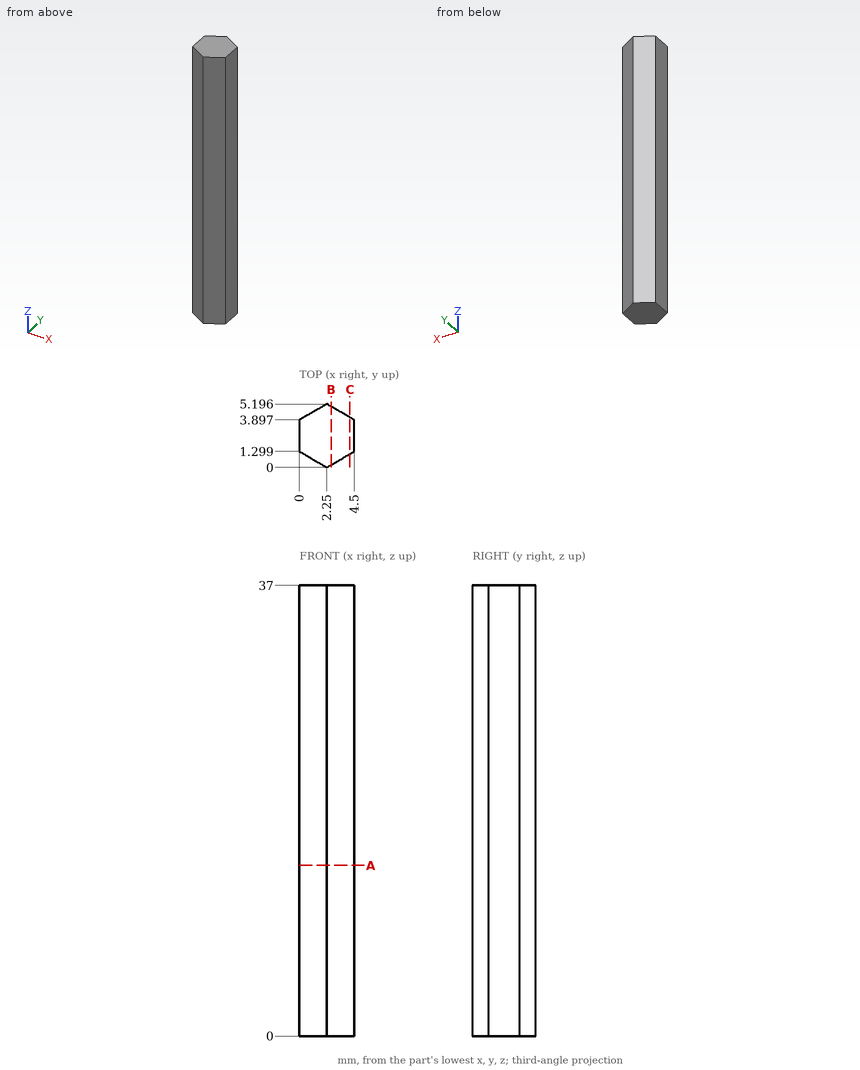
Could you check a few things on this drawing? It's one solid part, dimensions in mm from its lowest x, y, z. Round coordinates to 2 decimals unless told otherwise and drop trailing zeros. Order: outer loops, then holes, each group sorted by start corner. A loop starts at its lowest first (then second) coordinate and runs counter-clockwise, first axis right, second up. Notation, with made-up numbers: M 62,22.25 L 72,22.25 A5 ccw 72,27.25 Z; hole C 70.5,79 d9. An arc over 180 degrees is marked long. One line per item, written item: value.
(1) Imagine slicing it at B-B (x = 2.6). Write out the boundary of the cut face in (y, z), and give its area (3 significant figures).
Ans:
outline: M 0.2,0 L 4.99,0 L 4.99,37 L 0.2,37 Z
area: 177 mm^2
(2) Imagine slicing it at A-A (z = 14). Write out the boundary of the cut face in (x, y).
Ans:
outline: M 0,1.3 L 2.25,0 L 4.5,1.3 L 4.5,3.9 L 2.25,5.2 L 0,3.9 Z
(3) Imagine slicing it at C-C (x = 4.15). Write out the boundary of the cut face in (y, z), and give its area (3 significant figures).
Ans:
outline: M 1.1,0 L 4.1,0 L 4.1,37 L 1.1,37 Z
area: 111 mm^2
(4) I'm going to push a flat-ended pin straight in: P1, Ø1, axis at x = 1.5, z = 11, coming from the +Y side. Where does the tip first touch, or does it pass through?
Ans:
P1: stops at y = 5.05
(5) I need wall thicknesses on line 1 along Y through (x, z) = (3.4, 5); line 2 along X through (y, z) = (0.45, 23.5); line 3 along Y through (x, z) = (0.45, 9.5). Which ranges of each line are inside material? Lowest first, please. Write a range as from..to.
Ans:
line 1: y = 0.66..4.53
line 2: x = 1.47..3.03
line 3: y = 1.04..4.16
